from build123d import *

# Parameters (mm, degrees)
EXTRUDE_1_DEPTH     = 20
RIB_START           = -3
RIB_1_DEPTH         = 3
CUT_EXTRUDE_1_DEPTH = 42.952353927


# Read off the part's stored shape, not the designer's step: 筋1
with BuildPart() as part:
    # 草图1 → 拉伸-薄壁1 (new body)
    with BuildSketch(Plane(origin=(0, 0, 0), x_dir=(1, 0, 0), z_dir=(0, 1, 0))):
        Polygon((0, 28), (0, 0), (28, 0), (28, 4), (4, 4), (4, 28), align=None)
    extrude(amount=-EXTRUDE_1_DEPTH)

    # 筋1 outline → 筋1 (add)
    with BuildSketch(Plane(origin=(0, 0, 0), x_dir=(1, 0, 0), z_dir=(0, 1, 0)).offset(RIB_START)):
        Polygon((8, 28), (4, 28), (4, 4), (28, 4), (28, 8), (23, 8), (8, 23), align=None)
    rib_1 = extrude(amount=RIB_1_DEPTH)

    # 镜向1: 筋1 across plane
    add(rib_1.mirror(Plane(origin=(0, -10, 0), x_dir=(0, 0, 1), z_dir=(0, -1, 0))))

    # 草图3 → 切除-拉伸1 (cut, through all)
    with BuildSketch(Plane(origin=(4, 0, 0), x_dir=(0, 0, -1), z_dir=(1, 0, 0))):
        with BuildLine():
            Line((22, -13), (16, -13))
            ThreePointArc((16, -13), (13, -10), (16, -7))
            Line((16, -7), (22, -7))
            ThreePointArc((22, -7), (25, -10), (22, -13))
        make_face()
    cut_extrude_1 = extrude(amount=-CUT_EXTRUDE_1_DEPTH, mode=Mode.SUBTRACT)

    # 镜向2: 切除-拉伸1 across plane
    add(cut_extrude_1.mirror(Plane(origin=(0, 0, 0), x_dir=(-0.7071067811865478, 0, 0.7071067811865472), z_dir=(0.7071067811865475, 0, 0.7071067811865477))), mode=Mode.SUBTRACT)


solid = part.part
Could you check a few things on this model? Use its own coordinates, in mm. A direction names the side the tool comes from. Give positions to 0.01 mm unless a question says otherwise; leave off trailing zeros. Write each loop counter-clockwise with the first axis right and the second up, starting at its lowest first coordinate (ties: lowest second). Pieces come first, ordered by that corner, then holes. Notation, with made-up numbers: (-38.75, -11) - (-31.75, -11) arc R16 cw to (-31.75, 10) - close; hole circle Ø10 at (5.25, -1). An arc over 180 degrees is marked (long way). Use CSV: the item, a comma, the result in double quotes. Start each with the question number.
Item 1: I want a section at D-D, the plane x = 4.75. Please give me the cut outline in (y, z), then the cut area to 3 significant figures.
Item 2: I want a section at B-B, the plane x = 17.25. Please give me the cut outline in (y, z), then the cut area to 4 significant figures.
Item 3: I want a section at A-A, the plane z = -21.5. Please give me the cut outline in (x, y).
Item 4: I want a section at C-C, the plane y = -18. Please give me the cut outline in (x, z).
Item 5: For faces 1 (the face through (2, -10, -13)), 2 (the face through (13, -10, -2)), 3 (the face through (26, -18, -8)), 4 (the face through (10, -3, -14)), which set-ups out of +Z, -Z, +X, -X, +Y, -Y let a thin tool reach every point of the face, with its end or its side?
Item 6: If I drill on line 1 along Y through (x, z) = (12.5, -12); line 2 along X through (y, z) = (-4, -20); line 3 along Z through (x, y) = (4.5, -15), over which ranges is the centre line in solid material (lowest first)?
Item 7: I'm going to push flat-ended pins straight in: pin 1 (2 mm diameter, centred on y = -3, z = -20.5, fed in from +X); pin 2 (7 mm diameter, centred on x = 12, y = -12, fed in from -Z); pin 3 (0.9 mm diameter, centred on x = 25.5, y = -18, fed in from -Z); pin 4 (7 mm diameter, centred on x = 16, z = -21.5, fed in from -Y). Where does each tip first touch, or does it pass through?
Item 8: If we mould it in two halves opening along Y, with no side actions, what happens to faces 5 (the face through (2, -10, -25)), 6 (the face through (16.2, -6.8, -4)), 7 (the face through (28, -10, -3))? For each: pulls with the +Y half, pulls with the -Y half, needs draft (parallel to the pull), parting line crosses it, or undercut.
Findings:
1,outline,"(-20, -28) - (-17, -28) - (-17, -4) - (-3, -4) - (-3, -28) - (0, -28) - (0, 0) - (-20, 0) - close"
1,area,"224 mm2"
2,outline,"(-20, -13.75) - (-17, -13.75) - (-17, -4) - (-13, -4) - (-13, 0) - (-20, 0) - close; (-7, -4) - (-3, -4) - (-3, -13.75) - (0, -13.75) - (0, 0) - (-7, 0) - close"
2,area,"114.5 mm2"
3,outline,"(0, -20) - (9.5, -20) - (9.5, -17) - (4, -17) - (4, -13) - (0, -13) - close; (0, -7) - (4, -7) - (4, -3) - (9.5, -3) - (9.5, 0) - (0, 0) - close"
4,outline,"(0, -28) - (8, -28) - (8, -23) - (23, -8) - (28, -8) - (28, 0) - (0, 0) - close"
5,face 1,"+X, -X"
5,face 2,"+Z, -Z"
5,face 3,"-Z, +X, +Y, -Y"
5,face 4,"-Z, +X"
6,line 1,"y = -20 to -17, -3 to 0"
6,line 2,"x = 0 to 4"
6,line 3,"z = -4 to 0"
7,pin 1,"stops at x = 11.5"
7,pin 2,"stops at z = -4"
7,pin 3,"stops at z = -8"
7,pin 4,"passes through"
8,face 5,"undercut"
8,face 6,"undercut"
8,face 7,"needs draft"
